```python
from build123d import *

# Parameters (mm, degrees)
CYLINDER001_R           = 4.25
CYLINDER001_DEPTH       = 3.4
CYLINDER001_PITCH_ANGLE = 90
CYLINDER_R              = 2.7
CYLINDER_DEPTH          = 11
CYLINDER_PITCH_ANGLE    = 90
PAD001_DEPTH            = 8.5
SKETCH002_W             = 6
SKETCH002_H             = 1.5
POCKET_DEPTH            = 9.001
PAD_DEPTH               = 9.5
SKETCH003_R             = 3.25
POCKET001_DEPTH         = 3.4
SKETCH004_R             = 1.7
POCKET002_DEPTH         = 24.998848
SKETCH005_W             = 9
SKETCH005_H             = 14
PAD002_DEPTH            = 5


with BuildPart() as cylinder001:
    # Cylinder001 → Cylinder001 (new body)
    with BuildSketch(Plane.XY):
        Circle(CYLINDER001_R)
    extrude(amount=CYLINDER001_DEPTH)


with BuildPart() as cylinder001_1:
    # Cylinder001 pitch: moved
    add(cylinder001.part.rotate(Axis((0, 0, 0), (0, 1, 0)), CYLINDER001_PITCH_ANGLE))


with BuildPart() as cylinder001_2:
    # Cylinder001 placement: moved
    add(cylinder001_1.part.moved(Location((-13, -6, 0))))


with BuildPart() as screw_tube:
    # Cylinder → Cylinder (new body)
    with BuildSketch(Plane.XY):
        Circle(CYLINDER_R)
    extrude(amount=CYLINDER_DEPTH)


with BuildPart() as screw_tube_1:
    # Cylinder pitch: moved
    add(screw_tube.part.rotate(Axis((0, 0, 0), (0, 1, 0)), CYLINDER_PITCH_ANGLE))


with BuildPart() as screw_tube_2:
    # Cylinder placement: moved
    add(screw_tube_1.part.moved(Location((-12.6, -6, 0))))

    # Fusion: union Cylinder001
    add(cylinder001_2.part)


with BuildPart() as pocket:
    # Sketch001 → Pad001 (new body, symmetric)
    with BuildSketch(Plane.XY):
        with BuildLine():
            Line((-12, 0), (-12, -7.3))
            ThreePointArc((-12, -7.3), (-10.174376, -12.864965), (-5.407034, -16.267051))
            Line((-5.407034, -16.267051), (6.329406, -19.933783))
            Line((6.329406, -19.933783), (7.579268, -20.324269))
            Line((7.579268, -20.324269), (9.655694, -19.568512))
            Line((9.655694, -19.568512), (8.813242, -19.029741))
            Line((1.612292, -14.424542), (8.813242, -19.029741))
            ThreePointArc((-3, -6), (-1.771466, -10.802245), (1.612292, -14.424542))
            Line((-3, 0), (-3, -6))
            Line((-3, 1), (-3, 0))
            Line((-12, 1), (-3, 1))
            Line((-12, 0), (-12, 1))
        make_face()
    extrude(amount=PAD001_DEPTH, both=True)

    # Sketch002 → Pocket (cut, through all)
    with BuildSketch(Plane.YZ.offset(-3)):
        with Locations((-2, 7.75)):
            Rectangle(SKETCH002_W, SKETCH002_H)
        with Locations((-2, -7.75)):
            Rectangle(SKETCH002_W, SKETCH002_H)
    extrude(amount=-POCKET_DEPTH, mode=Mode.SUBTRACT)


with BuildPart() as top:
    # Sketch → Pad (new body, symmetric)
    with BuildSketch(Plane.XY):
        with BuildLine():
            Line((0, 0), (-15, 0))
            Line((-15, 0), (-15, -8))
            ThreePointArc((-15, -8), (-11.192388, -17.192388), (-2, -21))
            Line((-2, -21), (3.42, -21))
            Line((3.42, -21), (9.997848, -18.605859))
            Line((1.997848, -13.489646), (9.997848, -18.605859))
            ThreePointArc((0, -10), (0.5348, -12.010537), (1.997848, -13.489646))
            Line((0, 0), (0, -10))
        make_face()
    extrude(amount=PAD_DEPTH, both=True)

    # Cut: cut Pocket
    add(pocket.part, mode=Mode.SUBTRACT)

    # Fusion001: union screw-tube
    add(screw_tube_2.part)

    # Sketch003 → Pocket001 (cut)
    with BuildSketch(Plane(origin=(-15, 0, 0), x_dir=(0, -1, 0), z_dir=(-1, 0, 0))):
        with Locations((6, 0)):
            Circle(SKETCH003_R)
    extrude(amount=-POCKET001_DEPTH, mode=Mode.SUBTRACT)

    # Sketch004 → Pocket002 (cut, through all)
    with BuildSketch(Plane(origin=(-15, 0, 0), x_dir=(0, -1, 0), z_dir=(-1, 0, 0))):
        with Locations((6, 0)):
            Circle(SKETCH004_R)
    extrude(amount=-POCKET002_DEPTH, mode=Mode.SUBTRACT)

    # Sketch005 → Pad002 (new body)
    with BuildSketch(Plane(origin=(0, 0, 0), x_dir=(-1, 0, 0), z_dir=(0, 1, 0))):
        with BuildLine():
            ThreePointArc((3.25, 7.9), (2.18934, 7.46066), (1.75, 6.4))
            Line((1.75, 6.4), (1.75, -6.4))
            ThreePointArc((1.75, -6.4), (2.18934, -7.46066), (3.25, -7.9))
            Line((3.25, -7.9), (11.75, -7.9))
            ThreePointArc((11.75, -7.9), (12.81066, -7.46066), (13.25, -6.4))
            Line((13.25, 6.4), (13.25, -6.4))
            ThreePointArc((13.25, 6.4), (12.81066, 7.46066), (11.75, 7.9))
            Line((3.25, 7.9), (11.75, 7.9))
        make_face()
        with Locations((7.5, 0)):
            Rectangle(SKETCH005_W, SKETCH005_H, mode=Mode.SUBTRACT)
    extrude(amount=PAD002_DEPTH)


solid = top.part
```
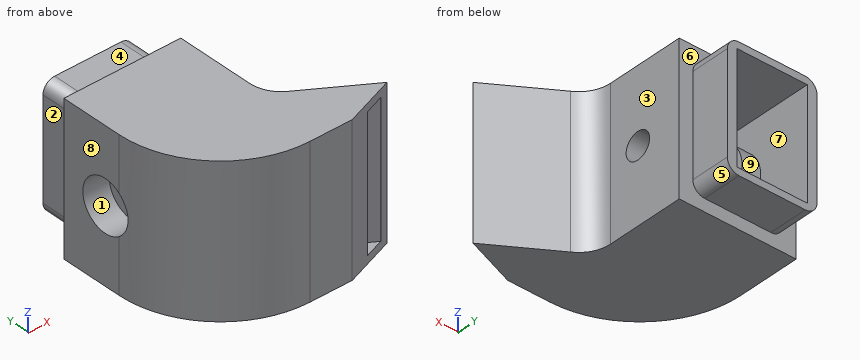
The listing builds one solid part. Answer for the finished solid, in the listing's coordinates (mm). Face numbers are marked on the shaded views. A direction names the side the tool comes from. Give positions to 0.01 mm unless a question says otherwise; leave off trailing zeros. Order: outer loops, then holes, each group sorted by start corner. A loop starts at its lowest first (then second) coordinate and runs counter-clockwise, first axis right, second up. Notation, with made-up numbers: M -20,-12 L 17,-12 A15 ccw 17,11 Z; hole C -22.5,-32 d5. An arc over 180 degrees is marked long. Put each result on its own line as item: value. Start each with the question number.
Item 1: The part is cut by section B-B, the plane x = -4.5. Determine the outline of the cut face in (y, z), and give its area (3 significant figures).
Item 2: Find the intervals of material crossed by line 1 along Z through (x, y) = (-7, -6); line 2 along Z through (x, y) = (-13.2, -6); line 3 along X through (y, z) = (-2.75, 4.75), in increasing order.
Item 3: The part is cut by section D-D, the plane x = 0.75. Determine the outline of the cut face in (y, z), and give its area (3 significant figures).
Item 4: Which of the six approach directions +Z, -Z, +X, -X, +Y, -Y give full straight-line access (tool end or side, diameter ignored) to the marked faces 1, 2, 3, 4 and 5?
Item 5: The part is cut by section A-A, the plane y = 1.5. Determine the outline of the cut face in (x, z), and give its area (3 significant figures).
Item 6: For a pull along X with two mould halves and no side action, classify the marked faces 6, 7, 8 and 9 as +X half, -X half, draft (parallel to the pull), parting line (faces both ways), or undercut.
Item 7: Flat-ended cylindrical pins translate along their axes: P1, Ø5, axis at y = -6, z = 0, coming from the +X side; P2, Ø1.5, axis at x = -10, z = -6, coming from the +Y side; P3, Ø5.5, axis at y = 3, z = 0, coming from the +X side. Find the tip coordinate at first contact, or state that the pin passes through.
Answer key:
1. outline: M -20.76,-9.5 L 0,-9.5 L 0,-7.9 L 5,-7.9 L 5,-7 L -5,-7 L -5,-8.5 L -16.55,-8.5 L -16.55,8.5 L -5,8.5 L -5,7 L 5,7 L 5,7.9 L 0,7.9 L 0,9.5 L -20.76,9.5 Z; C -6,0 d5.4; hole C -6,0 d3.4
1. area: 151 mm²
2. line 1: z = -9.5 to -8.5, -2.7 to -1.7, 1.7 to 2.7, 8.5 to 9.5
2. line 2: z = -9.5 to -3.25, 3.25 to 9.5
2. line 3: x = -15 to -12, -3 to 0
3. outline: M -21,-9.5 L -12.35,-9.5 L -12.35,9.5 L -21,9.5 Z; hole M -18.19,-8.5 L -13.81,-8.5 L -13.81,8.5 L -18.19,8.5 Z
3. area: 89.9 mm²
4. face 1: -X
4. face 2: +Z, -Z, -X, +Y
4. face 3: +Z, -Z, +X, +Y
4. face 4: +Z, +X, -X, +Y
4. face 5: -Z, +X, +Y
5. outline: M -13.25,-6.4 A1.5 ccw -11.75,-7.9 L -3.25,-7.9 A1.5 ccw -1.75,-6.4 L -1.75,6.4 A1.5 ccw -3.25,7.9 L -11.75,7.9 A1.5 ccw -13.25,6.4 Z; hole M -12,-7 L -3,-7 L -3,7 L -12,7 Z
5. area: 53.8 mm²
6. face 6: draft
6. face 7: undercut
6. face 8: -X half
6. face 9: undercut
7. P1: stops at x = 0
7. P2: stops at y = -11.98
7. P3: stops at x = -1.75
